Can you work these out from the drawing? Everything is in mm from the part's minimum corner. A direction names the side the tool comes from. Round coordinates to 2 decimals unless told otherwise and drop trailing zeros. Order: outer loops, then holes, each group sorted by start corner. A loop starts at its lowest first (then second) coordinate and runs counter-clockwise, first axis right, second up. Notation, with made-up numbers: M 67.25,51.25 L 95.25,51.25 A20 cw 95.25,60.25 Z; hole C -37.5,70.5 d3. An arc over 180 degrees is marked long. Write item = value, one per line. Start each with the question number.
Item 1: I want a section at D-D, the plane x = 25.4. List the corners of the cut face in (y, z) for me (3 decimals), plus the area to 3 significant figures.
Item 2: I want a section at C-C, the plane y = 30.48. List the corners of the cut face in (x, z) for me (3 decimals).
Item 3: For the marked faces 4 and 5, which set-ups out of +Z, -Z, +X, -X, +Y, -Y let a thin tool reach every point of the face, with its end or its side?
Item 4: Please list where these lines run through material, in increasing order: L1, parallel to Y at x = 6.35, z = 3.75 (3 decimals); L2, parallel to X at y = 43, z = 1.25; L3, parallel to X at y = 33.5, z = 5.25.
Item 5: I want a section at B-B, the plane x = 44.45. List the corners of the cut face in (y, z) for me (3 decimals), plus the area to 3 significant figures.
Item 6: We'd pull the mould along X, two halves only. Please class the marked faces 1, 2 and 3: pulls with the +X half, pulls with the -X half, needs draft (parallel to the pull), parting line crosses it, or undercut.
Item 7: I'm going to push flat-ended pins straight in: P1, Ø3, axis at y = 30.48, z = 6.35, coming from the +X side; P2, Ø5, axis at x = 34.5, y = 17.5, coming from the -Z side; P3, Ø3, axis at x = 25.4, z = 6.35, coming from the -Y side; P4, Ø1, axis at x = 7, y = 7, coming from the -Z side. Where does each tip first touch, or does it pass through?
Item 8: I want a section at A-A, the plane z = 6.35. State how many separate pieces and enclosed holes the cut face has, plus the area to 3 significant figures.
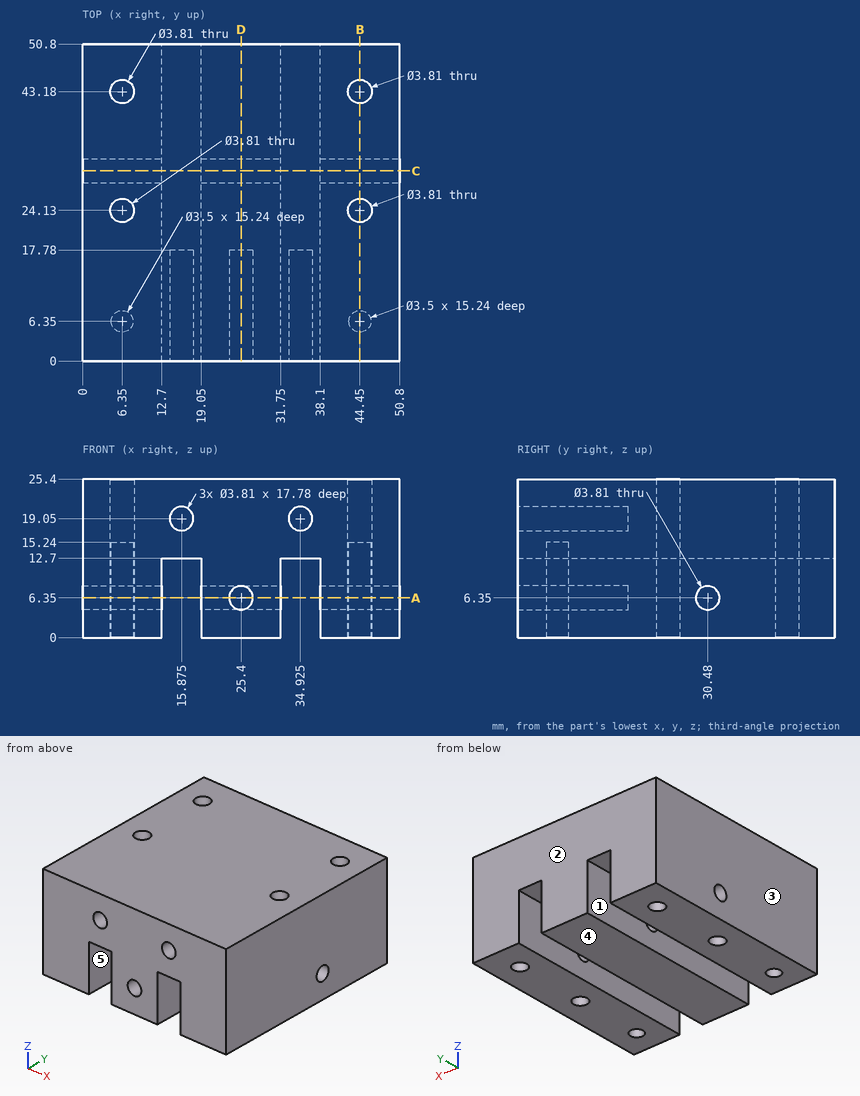
Filled in:
q1.outline = M 0,0 L 50.8,0 L 50.8,25.4 L 0,25.4 L 0,8.255 L 17.78,8.255 L 17.78,4.445 L 0,4.445 Z; hole C 30.48,6.35 d3.81
q1.area = 1,210 mm^2
q2.outline = M 0,0 L 12.7,0 L 12.7,4.445 L 0,4.445 Z; M 0,8.255 L 12.7,8.255 L 12.7,12.7 L 19.05,12.7 L 19.05,8.255 L 31.75,8.255 L 31.75,12.7 L 38.1,12.7 L 38.1,8.255 L 50.8,8.255 L 50.8,25.4 L 0,25.4 Z; M 19.05,0 L 31.75,0 L 31.75,4.445 L 19.05,4.445 Z; M 38.1,0 L 50.8,0 L 50.8,4.445 L 38.1,4.445 Z
q3.face_4 = -Z, +X, -X, +Y, -Y
q3.face_5 = -Z, +Y, -Y
q4.L1 = 0 to 4.6, 8.1 to 22.225, 26.035 to 41.275, 45.085 to 50.8
q4.L2 = 0 to 4.45, 8.25 to 12.7, 19.05 to 31.75, 38.1 to 42.55, 46.35 to 50.8
q4.L3 = 0 to 12.7, 19.05 to 31.75, 38.1 to 50.8
q5.outline = M 0,0 L 4.6,0 L 4.6,15.24 L 8.1,15.24 L 8.1,0 L 22.225,0 L 22.225,25.4 L 0,25.4 Z; M 26.035,0 L 41.275,0 L 41.275,25.4 L 26.035,25.4 Z; M 45.085,0 L 50.8,0 L 50.8,25.4 L 45.085,25.4 Z; hole C 30.48,6.35 d3.81
q5.area = 1,030 mm^2
q6.face_1 = undercut
q6.face_2 = needs draft
q6.face_3 = pulls with the -X half
q7.P1 = through
q7.P2 = 12.7
q7.P3 = 17.78
q7.P4 = 15.24
q8.separate_pieces = 6
q8.enclosed_holes = 6
q8.area = 1,660 mm^2
